```python
from build123d import *

# Parameters (mm, degrees)
BOSS_EXTRUDE2_DEPTH = 4.8
SKETCH4_W           = 2390
SKETCH4_H           = 1490
BOSS_EXTRUDE3_DEPTH = 447.4
BOSS_EXTRUDE4_DEPTH = 4.8


with BuildPart() as part:
    # Sketch1 → Boss-Extrude2 (new body)
    with BuildSketch(Plane(origin=(0, 0, 0), x_dir=(1, 0, 0), z_dir=(0, 1, 0))):
        with BuildLine():
            Line((-1190.348, -750), (1190.348, -750))
            ThreePointArc((1190.348, -750), (1197.172994652, -747.172994652), (1200, -740.348))
            Line((1200, -740.348), (1200, 740.348))
            ThreePointArc((1200, 740.348), (1197.172994652, 747.172994652), (1190.348, 750))
            Line((1190.348, 750), (-1190.348, 750))
            ThreePointArc((-1190.348, 750), (-1197.172994652, 747.172994652), (-1200, 740.348))
            Line((-1200, 740.348), (-1200, -740.348))
            ThreePointArc((-1200, -740.348), (-1197.172994652, -747.172994652), (-1190.348, -750))
        make_face()
    extrude(amount=-BOSS_EXTRUDE2_DEPTH)

    # Sketch4 → Boss-Extrude3 (add)
    with BuildSketch(Plane.XZ.offset(4.8)):
        Rectangle(SKETCH4_W, SKETCH4_H)
    extrude(amount=BOSS_EXTRUDE3_DEPTH)

    # Sketch5 → Boss-Extrude4 (add)
    with BuildSketch(Plane.XZ.offset(452.2)):
        with BuildLine():
            Line((1190.348, 750), (-1190.348, 750))
            ThreePointArc((-1190.348, 750), (-1197.172994652, 747.172994652), (-1200, 740.348))
            Line((-1200, 740.348), (-1200, -740.348))
            ThreePointArc((-1200, -740.348), (-1197.172994652, -747.172994652), (-1190.348, -750))
            Line((-1190.348, -750), (1190.348, -750))
            ThreePointArc((1190.348, -750), (1197.172994652, -747.172994652), (1200, -740.348))
            Line((1200, -740.348), (1200, 740.348))
            ThreePointArc((1200, 740.348), (1197.172994652, 747.172994652), (1190.348, 750))
        make_face()
    extrude(amount=BOSS_EXTRUDE4_DEPTH)


solid = part.part
```
Geometry check sheet. Reference: the model listing, model coordinates, mm. A direction names the side the tool comes from. Coordinates: 2 decimals unless noted, no trailing zeros. Answer as a JSON object with one key per item and string values. Group by question number.
Item 1: Draft check along Y on faces 4 (the face through (-17, -457, 10)), 5 (the face through (-17, -225, -745)), 6 (the face through (-17, 0, -11)). Enter one of: +Y half, -Y half, draft (parallel to the pull), parting line (faces both ways), or undercut.
Item 2: Scan lines: probe 1 along Z at (x, y) = (-1034.5, -71.5); probe 2 along X at (y, z) = (-277.5, -572). Record each from-to range of solid material in increasing order.
Item 3: Depth check by flat-ended pin: pin 1 Ø12 at (x, y) = (-820, -244.5) entering from +Z; pin 2 Ø2 at (x, y) = (349.5, -57.5) entering from -Z; pin 3 Ø4 at (y, z) = (-180.5, -222.5) entering from -X. Enter the tip coordinate at first touch or a pass-through.
Item 4: Tool access check on faces 1 (the face through (-17, -225, 745)), 2 (the face through (-1195, -225, -10)), 3 (the face through (1195, -225, -10)). Record the directions out of +Z, -Z, +X, -X, +Y, -Y that give a thin tool (end or side, any length) a straight path to the whole face; none if there is none.
Resolved:
{
 "1": {"face 4": "-Y half", "face 5": "undercut", "face 6": "+Y half"},
 "2": {"probe 1": "-745 to 745", "probe 2": "-1195 to 1195"},
 "3": {"pin 1": "z = 745", "pin 2": "z = -745", "pin 3": "x = -1195"},
 "4": {"face 1": "+Z, +X, -X", "face 2": "+Z, -Z, -X", "face 3": "+Z, -Z, +X"}
}
